Geometry: final body of the model. Coordinates: model frame, mm. A direction names the side the tool comes from. Round coordinates to 2 decimals unless told otherwise and drop trailing zeros. Order: outer loops, then holes, each group sorted by start corner. A loop starts at its lowest first (then second) coordinate and runs counter-clockwise, first axis right, second up. Notation, with made-up numbers: (-34, -27) -> (-27, -27) arc R26 ccw to (-27, -11) -> close; hole circle Ø1 at (-13, 31.5). An arc over 180 degrees is marked (long way). Put each result on its own line as item: value.
```python
from build123d import *

# Parameters (mm, degrees)
SKETCH001_W  = 12
SKETCH001_H  = 8
PAD001_DEPTH = 0.5
BOX001_W     = 0.5
BOX001_H     = 30
BOX001_DEPTH = 2
BOX_W        = 0.5
BOX_H        = 30
BOX_DEPTH    = 2
SKETCH002_R  = 3
PAD002_DEPTH = 5
SKETCH_W     = 60
SKETCH_H     = 18
SKETCH_R     = 0.9
SKETCH_R_2   = 0.5
PAD_DEPTH    = 10
FILLET_R     = 4
BOX002_W     = 65
BOX002_H     = 23
BOX002_DEPTH = 12


with BuildPart() as axle_retainer_cutout:
    # Sketch001 → Pad001 (new body)
    with BuildSketch(Plane.XY):
        with Locations((-20, 0)):
            Rectangle(SKETCH001_W, SKETCH001_H)
        with Locations((20, 0)):
            Rectangle(SKETCH001_W, SKETCH001_H)
    extrude(amount=PAD001_DEPTH)


with BuildPart() as axle2_cutouts:
    # Box001 → Box001 (new body)
    with BuildSketch(Plane(origin=(-22.25, -15, 0), x_dir=(1, 0, 0), z_dir=(0, 0, 1))):
        with Locations((0.25, 15)):
            Rectangle(BOX001_W, BOX001_H)
    extrude(amount=BOX001_DEPTH)


with BuildPart() as axle1_cutouts:
    # Box → Box (new body)
    with BuildSketch(Plane(origin=(21.75, -15, 0), x_dir=(1, 0, 0), z_dir=(0, 0, 1))):
        with Locations((0.25, 15)):
            Rectangle(BOX_W, BOX_H)
    extrude(amount=BOX_DEPTH)


with BuildPart() as cutouts:
    # Sketch002 → Pad002 (new body)
    with BuildSketch(Plane.XY):
        with Locations((-22, 5)):
            Circle(SKETCH002_R)
        with Locations((-22, -5)):
            Circle(SKETCH002_R)
        with Locations((22, 5)):
            Circle(SKETCH002_R)
        with Locations((22, -5)):
            Circle(SKETCH002_R)
    extrude(amount=PAD002_DEPTH)

    # Fusion: union axle_retainer_cutout, Axle2 cutouts, Axle1 cutouts
    add(axle_retainer_cutout.part)
    add(axle2_cutouts.part)
    add(axle1_cutouts.part)


with BuildPart() as fillet_body:
    # Sketch → Pad (new body)
    with BuildSketch(Plane.XY):
        Rectangle(SKETCH_W, SKETCH_H)
        with Locations((-18, 0)):
            Circle(SKETCH_R, mode=Mode.SUBTRACT)
        with Locations((18, 0)):
            Circle(SKETCH_R, mode=Mode.SUBTRACT)
        with Locations((-22, 0)):
            Circle(SKETCH_R_2, mode=Mode.SUBTRACT)
        with Locations((22, 0)):
            Circle(SKETCH_R_2, mode=Mode.SUBTRACT)
    extrude(amount=PAD_DEPTH)

    # Cut: cut Cutouts
    add(cutouts.part, mode=Mode.SUBTRACT)

    # Fillet
    fillet_edges = [fillet_body.edges().sort_by_distance(p)[0] for p in [
        (-30, -9, 5),
        (30, -9, 5),
        (30, 9, 5),
        (-30, 9, 5),
    ]]
    fillet(fillet_edges, radius=FILLET_R)


with BuildPart() as cut001:
    # Box002 → Box002 (new body)
    with BuildSketch(Plane(origin=(-32.5, -11.5, -2.5), x_dir=(1, 0, 0), z_dir=(0, 0, 1))):
        with Locations((32.5, 11.5)):
            Rectangle(BOX002_W, BOX002_H)
    extrude(amount=BOX002_DEPTH)

    # Cut001: cut Fillet body
    add(fillet_body.part, mode=Mode.SUBTRACT)


solid = cut001.part
```
1. Draft query along Y for faces 1 (the face through (-22, -5, 5)), 2 (the face through (18, 0, 9.5)). Return one class per face: +Y half, -Y half, draft (parallel to the pull), parting line (faces both ways), or undercut.
Ans:
face 1: undercut
face 2: draft
2. Set-up query: faces 3 (the face through (0, 9, 5)), 4 (the face through (-32.5, 0, 3)). Return all of +Z, -Z, +X, -X, +Y, -Y with unobstructed straight access to the full face (end or side cutting, diameter ignored); none if empty.
Ans:
face 3: +Z
face 4: +Z, -Z, -X, +Y, -Y
3. Material intervals for probe 1 along Y at (x, z) = (-12.5, 3.5); probe 2 along Y at (x, z) = (17.5, 4); probe 3 along X at (y, z) = (6.25, 1.5), sorted ascending.
Ans:
probe 1: -11.5 to -9, 9 to 11.5
probe 2: -11.5 to -9, -0.75 to 0.75, 9 to 11.5
probe 3: -32.5 to -29.8, -24.73 to -19.27, 19.27 to 24.73, 29.8 to 32.5
4. Cut plane B-B on x = -5. Return loops of the section in (y, z), and give its area (3 significant figures).
Ans:
outline: (-11.5, -2.5) -> (11.5, -2.5) -> (11.5, 9.5) -> (9, 9.5) -> (9, 0) -> (-9, 0) -> (-9, 9.5) -> (-11.5, 9.5) -> close
area: 105 mm²
5. Cut plane C-C on y = -6. Return loops of the section in (x, z), and give its area (3 significant figures).
Ans:
outline: (-32.5, -2.5) -> (32.5, -2.5) -> (32.5, 9.5) -> (29.87, 9.5) -> (29.87, 0) -> (24.83, 0) -> (24.83, 5) -> (19.17, 5) -> (19.17, 0) -> (-19.17, 0) -> (-19.17, 5) -> (-24.83, 5) -> (-24.83, 0) -> (-29.87, 0) -> (-29.87, 9.5) -> (-32.5, 9.5) -> close
area: 269 mm²
6. Contact query for flat-ended pins moving along their axis: P1, Ø5.5, axis at x = 10, y = -3, coming from the +Z side; P2, Ø3, axis at x = 21.5, y = 5, coming from the +Z side. Output: stop coordinate, or through.
Ans:
P1: z = 0
P2: z = 5
7. Cut plane A-A on z = 8.5. Return loops of the section in (x, y), and give its area (3 significant figures).
Ans:
outline: (-32.5, -11.5) -> (32.5, -11.5) -> (32.5, 11.5) -> (-32.5, 11.5) -> close; circle Ø1 at (-22, 0); circle Ø1.8 at (-18, 0); circle Ø1.8 at (18, 0); circle Ø1 at (22, 0); hole (-30, -5) arc R4 ccw to (-26, -9) -> (26, -9) arc R4 ccw to (30, -5) -> (30, 5) arc R4 ccw to (26, 9) -> (-26, 9) arc R4 ccw to (-30, 5) -> close
area: 435 mm²
8. Cut plane D-D on x = -18. Return loops of the section in (y, z).
Ans:
outline: (-11.5, -2.5) -> (11.5, -2.5) -> (11.5, 9.5) -> (9, 9.5) -> (9, 0) -> (4, 0) -> (4, 0.5) -> (0.9, 0.5) -> (0.9, 9.5) -> (-0.9, 9.5) -> (-0.9, 0.5) -> (-4, 0.5) -> (-4, 0) -> (-9, 0) -> (-9, 9.5) -> (-11.5, 9.5) -> close
